Read the model definition and answer for the solid it produces. Units are mm, in the model's axes. A direction names the side the tool comes from. Give positions to 0.01 mm unless a question says otherwise; leave off trailing zeros. Write each loop counter-clockwise with the first axis right and the second up, starting at its lowest first coordinate (ties: lowest second). Pieces come first, ordered by that corner, then holes. Notation, with made-up numbers: (34, 5) -> (45, 5) arc R24 ccw to (45, 38) -> close; hole circle Ø9 at (-20, 75.25). An arc over 180 degrees is marked (long way). Use a Markdown table: item, result.
from build123d import *

# Parameters (mm, degrees)
SKETCH1_W           = 45.5
SKETCH1_H           = 124.4
BOSS_EXTRUDE1_DEPTH = 1.2
SKETCH2_W           = 5
SKETCH2_H           = 8.185483871
CUT_EXTRUDE1_DEPTH  = 1.6
FILLET1_R           = 2
FILLET2_R           = 1
FILLET3_R           = 5


with BuildPart() as part:
    # Sketch1 → Boss-Extrude1 (new body)
    with BuildSketch(Plane.XY):
        with Locations((22.75, 62.2)):
            Rectangle(SKETCH1_W, SKETCH1_H)
    extrude(amount=BOSS_EXTRUDE1_DEPTH)

    # Sketch2 → Cut-Extrude1 (cut)
    with BuildSketch(Plane.XY.offset(1.2)):
        Polygon((7.25, 87.575), (12.25, 87.575), (12.25, 91.575), (3.25, 91.575), (3.25, 79.389516129), (7.25, 79.389516129), align=None)
        with Locations((9.75, 83.482258065)):
            Rectangle(SKETCH2_W, SKETCH2_H)
        Polygon((33.25, 79.389516129), (33.25, 87.575), (12.25, 87.575), (12.25, 79.389516129), (7.25, 79.389516129), (7.25, 45.010483871), (12.25, 45.010483871), (12.25, 36.825), (33.25, 36.825), (33.25, 45.010483871), (38.25, 45.010483871), (38.25, 79.389516129), align=None)
        with Locations((35.75, 83.482258065)):
            Rectangle(SKETCH2_W, SKETCH2_H)
        Polygon((42.25, 79.389516129), (42.25, 91.575), (33.25, 91.575), (33.25, 87.575), (38.25, 87.575), (38.25, 79.389516129), align=None)
        Polygon((42.25, 45.010483871), (38.25, 45.010483871), (38.25, 36.825), (33.25, 36.825), (33.25, 32.825), (42.25, 32.825), align=None)
        with Locations((35.75, 40.917741936)):
            Rectangle(SKETCH2_W, SKETCH2_H)
        Polygon((7.25, 36.825), (7.25, 45.010483871), (3.25, 45.010483871), (3.25, 32.825), (12.25, 32.825), (12.25, 36.825), align=None)
        with Locations((9.75, 40.917741936)):
            Rectangle(SKETCH2_W, SKETCH2_H)
    extrude(amount=-CUT_EXTRUDE1_DEPTH, mode=Mode.SUBTRACT)

    # Fillet1
    fillet1_edges = [part.edges().sort_by_distance(p)[0] for p in [
        (3.25, 79.389516129, 0.6),
        (12.25, 91.575, 0.6),
        (33.25, 91.575, 0.6),
        (42.25, 91.575, 0.6),
        (42.25, 79.389516129, 0.6),
        (38.25, 79.389516129, 0.6),
        (38.25, 45.010483871, 0.6),
        (42.25, 45.010483871, 0.6),
        (42.25, 32.825, 0.6),
        (33.25, 32.825, 0.6),
        (12.25, 32.825, 0.6),
        (3.25, 32.825, 0.6),
        (3.25, 45.010483871, 0.6),
        (7.25, 45.010483871, 0.6),
        (7.25, 79.389516129, 0.6),
        (3.25, 91.575, 0.6),
    ]]
    fillet(fillet1_edges, radius=FILLET1_R - 0.0001)  # a hair under: the kernel refuses the full size

    # Fillet2
    fillet2_edges = [part.edges().sort_by_distance(p)[0] for p in [
        (12.25, 36.825, 0.6),
        (12.25, 87.575, 0.6),
        (33.25, 87.575, 0.6),
        (33.25, 36.825, 0.6),
    ]]
    fillet(fillet2_edges, radius=FILLET2_R)

    # Fillet3
    fillet3_edges = [part.edges().sort_by_distance(p)[0] for p in [
        (0, 124.4, 0.6),
        (45.5, 124.4, 0.6),
        (45.5, 0, 0.6),
        (0, 0, 0.6),
    ]]
    fillet(fillet3_edges, radius=FILLET3_R)


solid = part.part
Item 1: A cutting plane is placed at B-B (y = 70.5). Give the vertices of the cut face in (x, z), then the cut area to 3 significant figures.
Return value:
| item | result |
|---|---|
| outline | (0, 0) -> (7.25, 0) -> (7.25, 1.2) -> (0, 1.2) -> close; (38.25, 0) -> (45.5, 0) -> (45.5, 1.2) -> (38.25, 1.2) -> close |
| area | 17.4 mm^2 |
Item 2: This flat-tipped pin is pushed along its axis until it touches: P1, Ø8, axis at x = 15, y = 79, coming from the -Z side. Where does it stop, or does it pass through?
Return value:
| item | result |
|---|---|
| P1 | through |
Item 3: A cutting plane is placed at A-A (x = 18.5). Give the vertices of the cut face in (y, z) (3 decimals), then the cut area to 3 significant figures.
Return value:
| item | result |
|---|---|
| outline | (0, 0) -> (36.825, 0) -> (36.825, 1.2) -> (0, 1.2) -> close; (87.575, 0) -> (124.4, 0) -> (124.4, 1.2) -> (87.575, 1.2) -> close |
| area | 88.4 mm^2 |
Item 4: Straight lines are drawn through the part: line 1 along Y through (x, z) = (35.5, 0.1) (3 decimals); line 2 along Y through (x, z) = (21, 1.1) (3 decimals); line 3 along X through (y, z) = (50.5, 0.4). For each, find the intervals that lie inside material, in ascending order. Write a range as [from, to].
Return value:
| item | result |
|---|---|
| line 1 | [0, 32.825], [91.575, 124.4] |
| line 2 | [0, 36.825], [87.575, 124.4] |
| line 3 | [0, 7.25], [38.25, 45.5] |
Item 5: For a pull along Y with two mould halves and no side action, classify faces 1 (the face through (1, 2, 1)), 2 (the face through (11.649, 33.395, 0.592)), 3 (the face through (3.82, 33.426, 0.592)), 4 (the face through (1.43, 122.9, 0.61)) as +Y half, -Y half, draft (parallel to the pull), parting line (faces both ways), or undercut.
Return value:
| item | result |
|---|---|
| face 1 | -Y half |
| face 2 | undercut |
| face 3 | undercut |
| face 4 | +Y half |
Item 6: A tool of negligible diameter and unlimited length cuts with its end or side. For faces 5 (the face through (3.85, 44.44, 0.59)), 6 (the face through (44, 122.97, 0.61)), from which of +Z, -Z, +X, -X, +Y, -Y can it reach the whole face along a straight path? Write none if from no direction.
Return value:
| item | result |
|---|---|
| face 5 | +Z, -Z |
| face 6 | +Z, -Z, +X, +Y |
